```python
from build123d import *

# Parameters (mm, degrees)
ESQUISSE1_W        = 100
ESQUISSE1_H        = 50
ESQUISSE1_R        = 1.6
BOSS_EXTRU_1_DEPTH = 1.6
ESQUISSE2_R        = 5
BOSS_EXTRU_2_DEPTH = 20
ESQUISSE3_W        = 17.40280045
ESQUISSE3_H        = 36.018530138
BOSS_EXTRU_3_DEPTH = 15


with BuildPart() as part:
    # Esquisse1 → Boss.-Extru.1 (new body)
    with BuildSketch(Plane.XY):
        Rectangle(ESQUISSE1_W, ESQUISSE1_H)
        with Locations((-46, 21)):
            Circle(ESQUISSE1_R, mode=Mode.SUBTRACT)
        with Locations((46, 21)):
            Circle(ESQUISSE1_R, mode=Mode.SUBTRACT)
        with Locations((46, -21)):
            Circle(ESQUISSE1_R, mode=Mode.SUBTRACT)
        with Locations((-46, -21)):
            Circle(ESQUISSE1_R, mode=Mode.SUBTRACT)
    extrude(amount=BOSS_EXTRU_1_DEPTH)

    # Esquisse2 → Boss.-Extru.2 (add)
    with BuildSketch(Plane.XY.offset(1.6)):
        with Locations((-42.277991317, 11.052639899)):
            Circle(ESQUISSE2_R)
        with Locations((-42.277991317, -11.052639899)):
            Circle(ESQUISSE2_R)
    extrude(amount=BOSS_EXTRU_2_DEPTH)

    # Esquisse3 → Boss.-Extru.3 (add)
    with BuildSketch(Plane.XY.offset(1.6)):
        with Locations((0.355180215, 3.481690573)):
            Rectangle(ESQUISSE3_W, ESQUISSE3_H)
    extrude(amount=BOSS_EXTRU_3_DEPTH)


solid = part.part
```
Here's how the part is built. I have some questions about the finished solid (model axes, mm). A direction names the side the tool comes from. Round coordinates to 2 decimals unless told otherwise and drop trailing zeros. Loops run counter-clockwise (first coordinate to the right, second up) from the corner with the lowest first, then second, coordinate; pieces in that order, holes last.
1. Thinking about a two-plate mould opening in Y: for faces 6 (the face through (9.057, 3, 9)), 7 (the face through (0, -14.528, 9)), 8 (the face through (-46.208, -19.414, 0.789)), which applies, released by +Y, released by -Y, zero draft, split by the parting line, or undercut?
Answers:
face 6: zero draft
face 7: released by -Y
face 8: undercut
2. Suppose I cut it at B-B, the plane y = -21. Please give me the cut outline in (x, z).
Answers:
outline: (-50, 0) - (-47.6, 0) - (-47.6, 1.6) - (-50, 1.6) - close; (-44.4, 0) - (44.4, 0) - (44.4, 1.6) - (-44.4, 1.6) - close; (47.6, 0) - (50, 0) - (50, 1.6) - (47.6, 1.6) - close
3. Suppose I cut it at D-D, the plane x = 8. Please give me the cut outline in (y, z), and give its area (3 significant figures).
Answers:
outline: (-25, 0) - (25, 0) - (25, 1.6) - (21.49, 1.6) - (21.49, 16.6) - (-14.53, 16.6) - (-14.53, 1.6) - (-25, 1.6) - close
area: 620 mm2
4. If I drill on probe 1 along Y at (x, z) = (-46, 0.45); probe 2 along Y at (x, z) = (-5, 10.5); probe 3 along Z at (x, y) = (11.5, -11), over which ranges is the centre line in solid material (lowest first)?
Answers:
probe 1: y = -25 to -22.6, -19.4 to 19.4, 22.6 to 25
probe 2: y = -14.53 to 21.49
probe 3: z = 0 to 1.6
5. Suppose I cut it at C-C, the plane z = 8.25. Please give me the cut outline in (x, y), and give its area (3 significant figures).
Answers:
outline: circle Ø10 at (-42.28, -11.05); circle Ø10 at (-42.28, 11.05); (-8.35, -14.53) - (9.06, -14.53) - (9.06, 21.49) - (-8.35, 21.49) - close
area: 784 mm2
6. Will these pins go through, and if not, where does the flat tip stop? pin 1 (6 mm diameter, centred on y = -7, z = 7.5, fed in from -X); pin 2 (5 mm diameter, centred on x = -4.5, y = -10, fed in from -Z); pin 3 (3 mm diameter, centred on x = 46, y = -21, fed in from +Z); pin 4 (5 mm diameter, centred on x = 0, y = 12.5, fed in from +Z).
Answers:
pin 1: stops at x = -47.17
pin 2: stops at z = 0
pin 3: passes through
pin 4: stops at z = 16.6
7. Suppose I cut it at A-A, the plane x = 46. Please give me the cut outline in (y, z), and give its area (3 significant figures).
Answers:
outline: (-25, 0) - (-22.6, 0) - (-22.6, 1.6) - (-25, 1.6) - close; (-19.4, 0) - (19.4, 0) - (19.4, 1.6) - (-19.4, 1.6) - close; (22.6, 0) - (25, 0) - (25, 1.6) - (22.6, 1.6) - close
area: 69.8 mm2
8. For faces 1 (the face through (-39.59, 15.27, 11.46)), 2 (the face through (-42, 11, 21.6)), 3 (the face through (0, 21.491, 9)), 4 (the face through (0, 4, 16.6)), 5 (the face through (-8.346, 3, 9)), which set-ups out of +Z, -Z, +X, -X, +Y, -Y let a thin tool reach every point of the face, with its end or its side?
Answers:
face 1: +Z
face 2: +Z, +X, -X, +Y, -Y
face 3: +Z, +X, -X, +Y
face 4: +Z, +X, +Y, -Y
face 5: +Z, +Y, -Y
